The model under review builds one solid part; all positions refer to its coordinate system, in mm. A direction names the side the tool comes from. Round coordinates to 2 decimals unless told otherwise and drop trailing zeros. Order: outer loops, then holes, each group sorted by start corner. A loop starts at its lowest first (then second) coordinate and runs counter-clockwise, first axis right, second up.
1) Consider section B-B (x = 0.75). Give the boundary of the cut face in (y, z), then the cut area to 3 significant figures.
2) Clearance check with flat-ended pins moving along their axes: P1, Ø3, axis at x = -3, y = -36.5, coming from the +Z side; P2, Ø3, axis at y = -30.5, z = 1.5, coming from the -X side; P3, Ø1.5, axis at x = 1.5, y = -37, coming from the +Z side; P4, Ø0.9, axis at y = 2, z = -0.5, coming from the -X side. State where each tip first meets the part, or that it passes through.
3) Consider section C-C (y = -42). Give the boundary of the cut face in (x, z).
4) Consider section A-A (z = 0). Give the boundary of the cut face in (x, y), then the cut area to 3 significant figures.
5) Machinability: for faces 4 (the face through (-0.9, -24.65, 2.86)), 5 (the face through (-1.257, 2.958, -2.219)), 6 (the face through (-2, 6, 2)), which of the approach directions +Z, -Z, +X, -X, +Y, -Y give a long, thin tool a straight path to every point of the face, cutting with its end or side? Answer none if there is none.
6) To check wall thickness, follow L1, parallel to Y at x = 3.25, z = 0; L2, parallel to Y at x = -2.25, z = 0.25; L3, parallel to Z at x = 1.5, y = 1. State the ranges of each line that lie inside material, in increasing order.
7) Consider section D-D (x = 4). Give the boundary of the cut face in (y, z), then the cut area to 3 significant figures.
8) Mouldability with a two-part tool opening along Z and no side actions: class faces 1 (the face through (1.29, 2.96, -2.2)), 2 (the face through (-3.3, 0, -0.1)), 3 (the face through (-4.88, 2.96, -1.08)) as pulls with the +Z half, pulls with the -Z half, needs draft (parallel to the pull), parting line crosses it, or undercut.
from build123d import *

# Parameters (mm, degrees)
SKETCH_1_R      = 5
EXTRUDE_1_DEPTH = 6
SKETCH_2_R      = 3
EXTRUDE_2_DEPTH = 50


with BuildPart() as part:
    # Эскиз1 → Вытянуть1 (new body)
    with BuildSketch(Plane(origin=(0, 0, 0), x_dir=(1, 0, 0), z_dir=(0, 1, 0))):
        with Locations(Location((0, 0, 0), (0, 0, 270))):
            Circle(SKETCH_1_R)
        Polygon((0, -2.944486373), (2.55, -1.472243186), (2.55, 1.472243186), (0, 2.944486373), (-2.55, 1.472243186), (-2.55, -1.472243186), align=None, mode=Mode.SUBTRACT)
    extrude(amount=EXTRUDE_1_DEPTH)

    # Эскиз2 → Вытянуть2 (add)
    with BuildSketch(Plane.XZ):
        with Locations(Location((0, 0, 0), (0, 0, 90))):
            Circle(SKETCH_2_R)
    extrude(amount=EXTRUDE_2_DEPTH)


solid = part.part
Answer below:
1. outline: (-50, -2.9) - (0, -2.9) - (0, -4.94) - (6, -4.94) - (6, -2.51) - (0, -2.51) - (0, 2.51) - (6, 2.51) - (6, 4.94) - (0, 4.94) - (0, 2.9) - (-50, 2.9) - close
1. area: 320 mm2
2. P1: stops at z = 2.6
2. P2: stops at x = -3
2. P3: stops at z = 2.9
2. P4: stops at x = -5
3. outline: circle Ø6 at (0, 0)
4. outline: (-5, 0) - (-3, 0) - (-3, -50) - (3, -50) - (3, 0) - (5, 0) - (5, 6) - (2.55, 6) - (2.55, 0) - (-2.55, 0) - (-2.55, 6) - (-5, 6) - close
4. area: 329 mm2
5. face 4: -Y
5. face 5: +Y
5. face 6: +Z, -Z, +X, -X, +Y
6. L1: y = 0 to 6
6. L2: y = -50 to 0
6. L3: z = -4.77 to -2.08, 2.08 to 4.77
7. outline: (0, -3) - (6, -3) - (6, 3) - (0, 3) - close
7. area: 36.0 mm2
8. face 1: undercut
8. face 2: needs draft
8. face 3: parting line crosses it
